Can you work these out from the drawing? Everything is in mm from the part's minimum corner. A direction names the side the tool comes from. Round coordinates to 2 decimals unless told otherwise and drop trailing zeros. Loops run counter-clockwise (first coordinate to the right, second up) from the corner with the lowest first, then second, coordinate; pieces in that order, holes last. Notation, with made-up numbers: (10.25, -15.5) - (62.25, -15.5) arc R34 cw to (62.25, 15.5) - close; hole circle Ø7 at (2.5, -12). An arc over 180 degrees is marked (long way). Return JSON: item names as keys, results as strings. Group by question number.
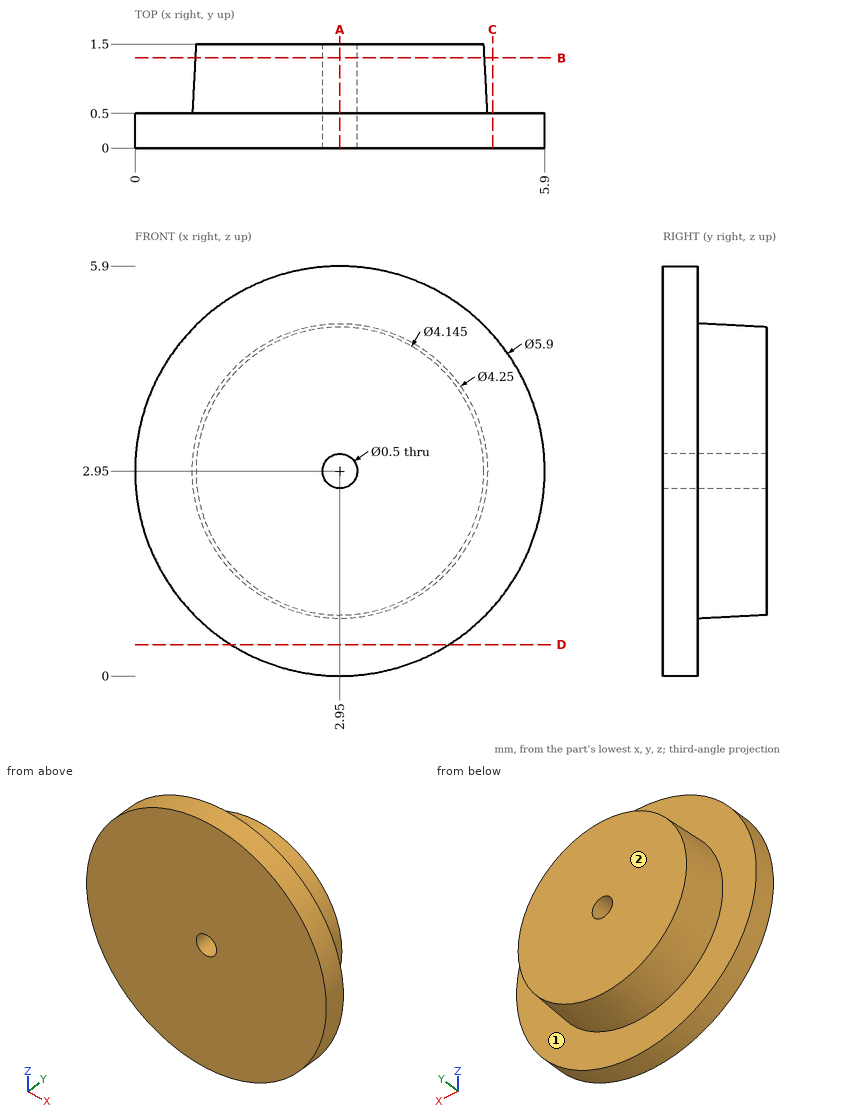
Q1. For the marked faces 1 and 2, which set-ups out of +Z, -Z, +X, -X, +Y, -Y let a thin tool reach every point of the face, with its end or its side?
Q2. Imagine slicing it at C-C, the plane x = 5.15. List the corners of the cut face in (y, z) for me (1 decimal).
Q3. Imagine slicing it at B-B, the plane y = 1.3. List the corners of the cut face in (x, z) for me, and give its area (3 significant figures).
Q4. Imagine slicing it at D-D, the plane z = 0.45. List the corners of the cut face in (x, y) for me.
Q5. Imagine slicing it at A-A, the plane x = 2.95. List the corners of the cut face in (y, z) for me (1 decimal).
Q6. Please list where these lines run through material, in increasing order: line 1 (X direction, y = 0.35, z = 2.95); line 2 (Y direction, x = 1.8, z = 5); line 3 (X direction, y = 1.1, z = 2.95).
Output values:
{
 "1": {"face 1": "+Y", "face 2": "+Z, -Z, +X, -X, +Y"},
 "2": {"outline": "(0, 1) - (0.5, 1) - (0.5, 4.9) - (0, 4.9) - close"},
 "3": {"outline": "circle Ø4.17 at (2.95, 2.95); hole circle Ø0.5 at (2.95, 2.95)", "area": "13.4 mm^2"},
 "4": {"outline": "(1.38, 0) - (4.52, 0) - (4.52, 0.5) - (1.38, 0.5) - close"},
 "5": {"outline": "(0, 0) - (0.5, 0) - (0.5, 0.8) - (1.5, 0.9) - (1.5, 2.7) - (0, 2.7) - close; (0, 3.2) - (1.5, 3.2) - (1.5, 5) - (0.5, 5.1) - (0.5, 5.9) - (0, 5.9) - close"},
 "6": {"line 1": "x = 0 to 2.7, 3.2 to 5.9", "line 2": "y = 0 to 0.5", "line 3": "x = 0.86 to 2.7, 3.2 to 5.04"}
}
